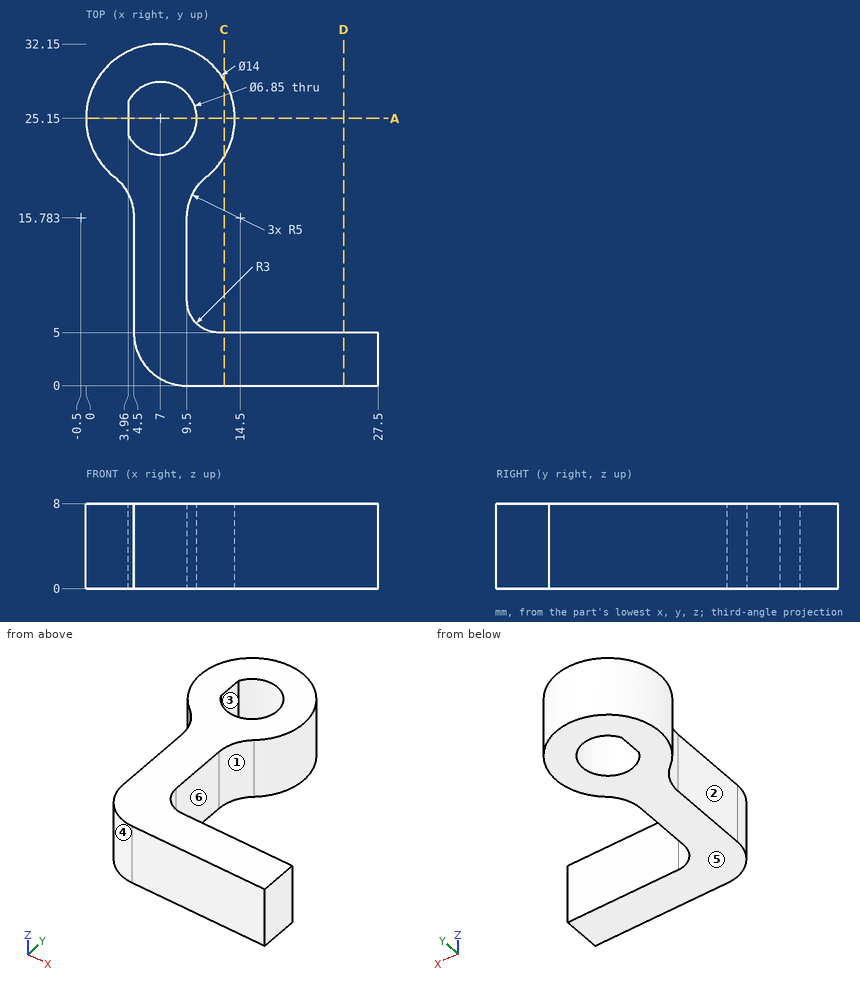
The figure shows three views and two pictorial views of one solid part (mm, origin at its lowest corner). Answer the questions. A direction names the side the tool comes from. Coordinates: 2 decimals unless noted, no trailing zeros. Loops run counter-clockwise (first coordinate to the right, second up) from the corner with the lowest first, then second, coordinate; pieces in that order, holes last. Notation, with made-up numbers: M 59.25,26.25 L 75.25,26.25 A17 cw 75.25,34.25 Z; hole C 18.5,85.5 d9. An arc over 180 degrees is marked long. Use CSV: the item, a comma, the result in double quotes. Start each with the question number.
(1) Given pin 1 Ø3.5 at (y, z) = (24.5, 6) entering from +X; pin 2 Ø3 at (x, z) = (24.5, 3) entering from +Y; pin 3 Ø10 at (x, y) = (6.5, 25.5) entering from +Z, each flat-ended and moving along its own axis, determine where each tip first touches the part or whether it passes through.
(2) Find section C-C, the plane x = 13. Give the vertices of the cut face in (y, z) (1 decimal).
(3) For the marked faces 1, 2 and 3, determine the directions among +Z, -Z, +X, -X, +Y, -Y from which every point of the face is accessible in a straight line to the end or side of a thin tool.
(4) Consider line 1 (Y direction, x = 25.75, z = 2.75); line 2 (X direction, y = 12, z = 4.25); line 3 (X direction, y = 24, z = 5.5) (1 decimal). Determine where each line is inside the solid, lowest interval first.
(5) Find section A-A, the plane y = 25.15. Give the vertices of the cut face in (x, z) (1 decimal).
(6) For a pull along Y with two mould halves and no side action, classify the marked faces 4, 5 and 6 as +Y half, -Y half, draft (parallel to the pull), parting line (faces both ways), or undercut.
(7) Find section D-D, the plane x = 24.25. Give the vertices of the cut face in (y, z), then the cut area to 3 significant figures.
Recorded:
1,pin 1,"stops at x = 14"
1,pin 2,"stops at y = 5"
1,pin 3,"stops at z = 8"
2,outline,"M 0,0 L 5,0 L 5,8 L 0,8 Z; M 21.5,0 L 28.8,0 L 28.8,8 L 21.5,8 Z"
3,face 1,"+Z, -Z, +X"
3,face 2,"+Z, -Z, -X, -Y"
3,face 3,"+Z, -Z"
4,line 1,"y = 0 to 5"
4,line 2,"x = 4.5 to 9.5"
4,line 3,"x = 0.1 to 4, 10.2 to 13.9"
5,outline,"M 0,0 L 4,0 L 4,8 L 0,8 Z; M 10.4,0 L 14,0 L 14,8 L 10.4,8 Z"
6,face 4,"-Y half"
6,face 5,"draft"
6,face 6,"undercut"
7,outline,"M 0,0 L 5,0 L 5,8 L 0,8 Z"
7,area,"40.0 mm^2"
